Check sheet for the modelled part. Datum: model origin and axes. Units: mm. Coordinates: 2 decimals unless noted, no trailing zeros. Write each loop counter-clockwise with the first axis right and the second up, starting at its lowest first coordinate (ties: lowest second). Pieces come first, ordered by that corner, then holes. Notation, with made-up numbers: (-34.5, 67.25) - (7.5, 67.25) arc R10 ccw to (7.5, 84.25) - close; hole circle Ø8 at (29.25, 58). An arc over 180 degrees is marked (long way). Use one line per item in the form item = value. Start each with the question number.
1. Cross-section at C-C on y = 88. Record the boundary of the cut face in (x, z), then the cut area to 3 significant figures.
2. Cross-section at A-A on y = 27. Record the boundary of the cut face in (x, z).
3. Scan lines: line 1 along Y through (x, z) = (4.5, 0.1); line 2 along Y through (x, z) = (-2.5, -0.05); line 3 along Y through (x, z) = (-0.5, 0.3). Record each from-to range of solid material in increasing order.
4. Cross-section at B-B on z = -0.7. Give the number of separate pieces and of enclosed holes in the cut face, then the cut area to 3 significant figures.
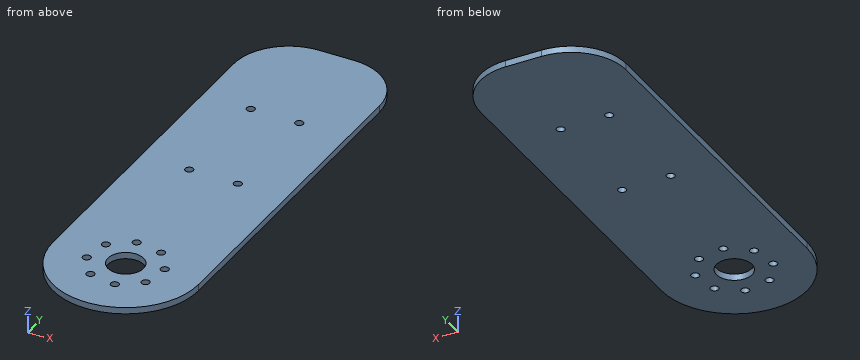
```python
from build123d import *

# Parameters (mm, degrees)
RESSALTO_EXTRUS_O1_DEPTH = 1
ESBO_O2_R                = 5.5
CORTE_EXTRUS_O1_DEPTH    = 101.189819842
ESBO_O3_R                = 1.25
CORTE_EXTRUS_O2_DEPTH    = 101.189819842
ESBO_O8_R                = 1.25
CORTE_EXTRUS_O3_DEPTH    = 17


with BuildPart() as part:
    # Esboço1 → Ressalto-extrusão1 (new, symmetric)
    with BuildSketch(Plane.XY):
        with BuildLine():
            Line((-25, -23), (-25, 80))
            ThreePointArc((-25, 80), (-20.02081528, 92.02081528), (-8, 97))
            Line((-8, 97), (3, 97))
            ThreePointArc((3, 97), (15.02081528, 92.02081528), (20, 80))
            Line((20, 80), (20, -23))
            ThreePointArc((20, -23), (-2.5, -45.5), (-25, -23))
        make_face()
    extrude(amount=RESSALTO_EXTRUS_O1_DEPTH, both=True)

    # Esboço2 → Corte-extrusão1 (cut, through all)
    with BuildSketch(Plane(origin=(0, 0, -1), x_dir=(-1, 0, 0), z_dir=(0, 0, -1))):
        with Locations((2.5, -23)):
            Circle(ESBO_O2_R)
    extrude(amount=-CORTE_EXTRUS_O1_DEPTH, mode=Mode.SUBTRACT)

    # Esboço3 → Corte-extrusão2 (cut, through all)
    with BuildSketch(Plane(origin=(0, 0, -1), x_dir=(-1, 0, 0), z_dir=(0, 0, -1))):
        with Locations((0.062167861, -33.726461414)):
            Circle(ESBO_O3_R)
        with Locations((-6.808561241, -28.860945967)):
            Circle(ESBO_O3_R)
        with Locations((-8.226461414, -20.562167861)):
            Circle(ESBO_O3_R)
        with Locations((-3.360945967, -13.691438759)):
            Circle(ESBO_O3_R)
        with Locations((4.937832139, -12.273538586)):
            Circle(ESBO_O3_R)
        with Locations((11.808561241, -17.139054033)):
            Circle(ESBO_O3_R)
        with Locations((13.226461414, -25.437832139)):
            Circle(ESBO_O3_R)
        with Locations((8.360945967, -32.308561241)):
            Circle(ESBO_O3_R)
    extrude(amount=-CORTE_EXTRUS_O2_DEPTH, mode=Mode.SUBTRACT)

    # Esboço8 → Corte-extrusão3 (cut)
    with BuildSketch(Plane.XY.offset(1)):
        with Locations((-10, 62)):
            Circle(ESBO_O8_R)
        with Locations((-10, 27)):
            Circle(ESBO_O8_R)
        with Locations((5, 62)):
            Circle(ESBO_O8_R)
        with Locations((5, 27)):
            Circle(ESBO_O8_R)
    extrude(amount=-CORTE_EXTRUS_O3_DEPTH, mode=Mode.SUBTRACT)


solid = part.part
```
Final values:
q1.outline = (-23, -1) - (18, -1) - (18, 1) - (-23, 1) - close
q1.area = 82.0 mm²
q2.outline = (-25, -1) - (-11.25, -1) - (-11.25, 1) - (-25, 1) - close; (-8.75, -1) - (3.75, -1) - (3.75, 1) - (-8.75, 1) - close; (6.25, -1) - (20, -1) - (20, 1) - (6.25, 1) - close
q3.line_1 = -44.38 to -14.21, -13.18 to 25.85, 28.15 to 60.85, 63.15 to 96.93
q3.line_2 = -45.5 to -28.5, -17.5 to 97
q3.line_3 = -45.41 to -34.9, -32.56 to -28.12, -17.88 to 97
q4.separate_pieces = 1
q4.enclosed_holes = 13
q4.area = 5,920 mm²
